Input: part model. Units: mm. Frame: model coordinates. Face numbers are marked on the shaded views. Give positions to 0.01 mm unless a question says otherwise; leave off trailing zeros. Loops run counter-clockwise (first coordinate to the right, second up) from the corner with the lowest first, then second, coordinate; pieces in that order, holes last. Notation, with made-up numbers: M 35,88 L 92,88 A24 ccw 92,123 Z; hole C 8.5,34.5 d10. An arc over 180 degrees is marked long. One line per item, written item: value. Start each with the question number.
(1) Section C-C on y = 1.3. Output: boundary loops of the cut face in (x, z) (3 decimals), plus the area to 3 significant figures.
(2) Section B-B on x = 0. Output: boundary loops of the cut face in (y, z), plus the area to 3 significant figures.
(3) Pull-direction query (Z, two-part tool) for the marked faces 1 and 2; classes: released by +Z, released by -Z, zero draft, split by the parting line, or undercut.
(4) Section D-D on z = -9. Output: boundary loops of the cut face in (x, y).
(5) Pin query (flat end, axial travel): P1, Ø2, axis at x = 5.5, z = -9, coming from the -Y side; P2, Ø1.3, axis at x = -5.5, z = -9, coming from the +Y side; P3, Ø1, axis at y = 4, z = 8.5, coming from the +X side. Return the tip coordinate at first contact, or that it passes through.
(6) Section A-A on y = 4.55. Output: boundary loops of the cut face in (x, z).
(7) Ray query, line 1 along X through (y, z) = (2.95, -9); line 2 along Z through (x, y) = (5.5, 3.95); line 3 along Y through (x, z) = (8.25, 10.25). Return the intervals inside material, ascending. Write a range as from..to.
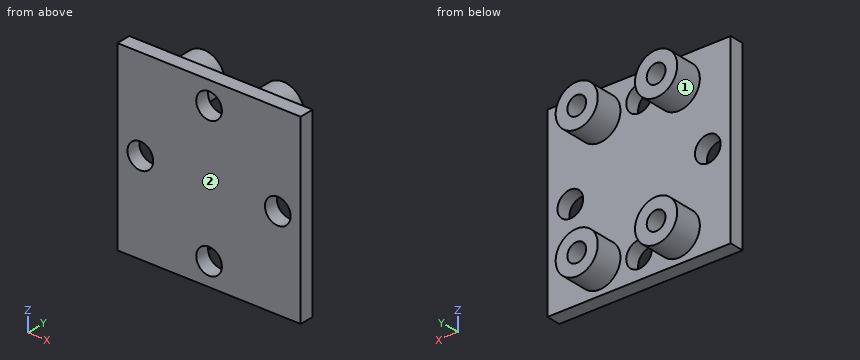
```python
from build123d import *

# Parameters (mm, degrees)
SKETCH1_W           = 25.4
SKETCH1_H           = 25.4
BOSS_EXTRUDE1_DEPTH = 2
SKETCH4_R           = 1.778
CUT_EXTRUDE1_DEPTH  = 3
SKETCH3_R           = 2.921
SKETCH3_R_2         = 1.3
BOSS_EXTRUDE2_DEPTH = 3.81
CIRPATTERN2_COUNT   = 4


with BuildPart() as part:
    # Sketch1 → Boss-Extrude1 (new body)
    with BuildSketch(Plane(origin=(0, 0, 0), x_dir=(1, 0, 0), z_dir=(0, 1, 0))):
        Rectangle(SKETCH1_W, SKETCH1_H)
    extrude(amount=BOSS_EXTRUDE1_DEPTH)

    # Sketch4 → Cut-Extrude1 (cut, through all)
    with BuildSketch(Plane(origin=(0, 0, 0), x_dir=(1, 0, 0), z_dir=(0, 1, 0))):
        with Locations((-9.525, 0)):
            Circle(SKETCH4_R)
    cut_extrude1 = extrude(amount=CUT_EXTRUDE1_DEPTH, mode=Mode.SUBTRACT)

    # Sketch3 → Boss-Extrude2 (add)
    with BuildSketch(Plane(origin=(0, 2, 0), x_dir=(1, 0, 0), z_dir=(0, 1, 0))):
        with Locations((-5.5, 9)):
            Circle(SKETCH3_R)
        with Locations((-5.5, 9)):
            Circle(SKETCH3_R_2, mode=Mode.SUBTRACT)
        with Locations((5.5, 9)):
            Circle(SKETCH3_R)
        with Locations((5.5, 9)):
            Circle(SKETCH3_R_2, mode=Mode.SUBTRACT)
        with Locations((5.5, -9)):
            Circle(SKETCH3_R)
        with Locations((5.5, -9)):
            Circle(SKETCH3_R_2, mode=Mode.SUBTRACT)
        with Locations((-5.5, -9)):
            Circle(SKETCH3_R)
        with Locations((-5.5, -9)):
            Circle(SKETCH3_R_2, mode=Mode.SUBTRACT)
    extrude(amount=BOSS_EXTRUDE2_DEPTH)

    # CirPattern2: Cut-Extrude1 ×4 about axis
    cirpattern2_axis = Axis((0, 0, 0), (0, 1, 0))
    for i in range(1, CIRPATTERN2_COUNT):
        add(cut_extrude1.rotate(cirpattern2_axis, i * 360 / CIRPATTERN2_COUNT), mode=Mode.SUBTRACT)


solid = part.part
```
Output values:
1. outline: M -12.7,-12.7 L 12.7,-12.7 L 12.7,12.7 L -12.7,12.7 Z; hole C -9.525,0 d3.556; hole C 0,-9.525 d3.556; hole C 0,9.525 d3.556; hole C 9.525,0 d3.556
1. area: 605 mm²
2. outline: M 0,-12.7 L 2,-12.7 L 2,-11.3 L 0,-11.3 Z; M 0,-7.75 L 2,-7.75 L 2,7.75 L 0,7.75 Z; M 0,11.3 L 2,11.3 L 2,12.7 L 0,12.7 Z
2. area: 36.6 mm²
3. face 1: undercut
3. face 2: zero draft
4. outline: M -12.7,0 L -1.7,0 L -1.7,2 L -2.58,2 L -2.58,5.81 L -4.2,5.81 L -4.2,2 L -6.8,2 L -6.8,5.81 L -8.42,5.81 L -8.42,2 L -12.7,2 Z; M 1.7,0 L 12.7,0 L 12.7,2 L 8.42,2 L 8.42,5.81 L 6.8,5.81 L 6.8,2 L 4.2,2 L 4.2,5.81 L 2.58,5.81 L 2.58,2 L 1.7,2 Z
5. P1: stops at y = 0
5. P2: stops at y = 2
5. P3: stops at x = 8.42
6. outline: C -5.5,-9 d5.84; C -5.5,9 d5.84; C 5.5,-9 d5.84; C 5.5,9 d5.84; hole C -5.5,-9 d2.6; hole C -5.5,9 d2.6; hole C 5.5,-9 d2.6; hole C 5.5,9 d2.6
7. line 1: x = -8.42..-6.8, -4.2..-2.58, 2.58..4.2, 6.8..8.42
7. line 2: z = -11.92..-10.3, -7.7..-6.08, 6.08..7.7, 10.3..11.92
7. line 3: y = 0..2
